The model under review builds one solid part; all positions refer to its coordinate system, in mm. Give positions to 0.01 mm unless a question says otherwise; leave off trailing zeros. Write each loop counter-clockwise with the first axis right and the second up, starting at its lowest first coordinate (ties: lowest second). Pieces come first, ordered by that corner, then holes. Notation, with made-up numbers: (47, -27.75) -> (65, -27.75) arc R31 ccw to (65, -0.75) -> close; hole circle Ø3 at (76, 66.5). An arc over 180 degrees is marked (long way). Use CSV: the item, a comma, the result in double quotes.
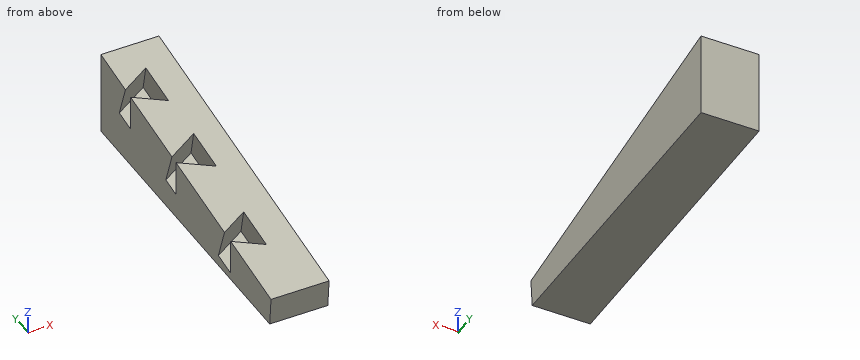
```python
from build123d import *

# Parameters (mm, degrees)
F1_DEPTH = 50.8
F3_DEPTH = 30.48
F3_TAPER = -8


with BuildPart() as f1:
    # F0 (on Right) → F1 (new body)
    with BuildSketch(Plane.YZ):
        Polygon((-134.3647271911, -22.5492262361), (-132.2128937073, -47.857912742), (147.1871062927, -47.857912742), (147.1871062927, 26.385902432), align=None)
    extrude(amount=F1_DEPTH)

    # F2 (on face) → F3 (cut)
    with BuildSketch(Plane(origin=(0, -0.1356486827, 0.780464594), x_dir=(1, 0, 0), z_dir=(0, -0.1712378928, 0.9852297113))):
        Polygon((23.9652451582, -44.2607051253), (0, -58.0970458686), (0, -68.524364382), (23.9652451582, -82.3607051253), align=None)
        Polygon((25.5085083311, 123.0692242943), (0, 108.3418801427), (0, 99.6965684458), (25.5085083311, 84.9692242943), align=None)
        Polygon((27.1452323874, 45.8107569695), (0, 30.1384497434), (0, 23.3830641955), (27.1452323874, 7.7107569695), align=None)
    extrude(amount=-F3_DEPTH, taper=F3_TAPER, mode=Mode.SUBTRACT)


solid = f1.part
```
Q1. Consider section A-A (x = 44). Write out the cut boundary in (y, z).
Derived:
outline,"(-134.36, -22.55) -> (-132.21, -47.86) -> (147.19, -47.86) -> (147.19, 26.39) -> close"
Q2. Insertion check: pin 1 (10 mm diameter, centred on x = 27, y = 118, fed in from +Z); pin 2 (6 mm diameter, centred on x = 43, y = -72.5, fed in from +Z). Each pin has a flat end and moves straight along its axis. Give the tip position at first contact, or say it passes through.
Derived:
pin 1,"stops at z = 22.18"
pin 2,"stops at z = -11.28"
Q3. Consider section B-B (y = 63.5). Write out the cut boundary in (x, z), then the cut area to 3 significant figures.
Derived:
outline,"(0, -47.86) -> (50.8, -47.86) -> (50.8, 11.84) -> (0, 11.84) -> close"
area,"3,030 mm2"
Q4. To check wall thickness, follow probe 1 along Y at (x, z) = (11, 5.5); probe 2 along X at (y, z) = (130, -0.5); probe 3 along Y at (x, z) = (23, -30). State the ranges of each line that lie inside material, in increasing order.
Derived:
probe 1,"y = 36.34 to 91.96, 118.02 to 147.19"
probe 2,"x = 0 to 27.42, 28.82 to 50.8"
probe 3,"y = -133.73 to -80.54, -36.3 to 147.19"
